```python
from build123d import *
from OCP.BRepFilletAPI import BRepFilletAPI_MakeChamfer

# Parameters (mm, degrees)
ESBO_O10_W               = 40
ESBO_O10_H               = 17.5
RESSALTO_EXTRUS_O6_DEPTH = 1.5
CORTE_EXTRUS_O2_DEPTH    = 2.5
ESBO_O12_W               = 3.5
ESBO_O12_H               = 2.75
RESSALTO_EXTRUS_O7_DEPTH = 1.2
ESBO_O13_W               = 3
ESBO_O13_H               = 1.5
ESBO_O13_W_2             = 2
CORTE_EXTRUS_O3_DEPTH    = 8
CORTE_EXTRUS_O4_DEPTH    = 20
CHANFRO5_SIZE            = 6
CHANFRO5_SIZE_2          = 0.419560872
CHANFRO6_SIZE            = 1
CHANFRO6_SIZE2           = 0.839099631
FILETE1_R                = 2


with BuildPart() as part:
    # Esboço10 → Ressalto-extrusão6 (new body)
    with BuildSketch(Plane.XY):
        Rectangle(ESBO_O10_W, ESBO_O10_H)
    extrude(amount=RESSALTO_EXTRUS_O6_DEPTH)

    # Esboço11 → Corte-extrusão2 (cut)
    with BuildSketch(Plane.XY.offset(1.5)):
        Polygon((-20, 3.75), (-15.75, 3.75), (-15.75, 8.75), (-12.25, 8.75), (-12.25, 3.75), (-3.75, 3.75), (-3.75, 9.75), (3.75, 9.75), (3.75, 3.75), (12.25, 3.75), (12.25, 8.75), (15.75, 8.75), (15.75, 3.75), (20, 3.75), (20, 11.902365005), (-20, 11.902365005), align=None)
        Polygon((-20, -4.25), (-15.75, -4.25), (-15.75, -8.75), (-12.25, -8.75), (-12.25, -4.25), (-3.75, -4.25), (-3.75, -10.25), (3.75, -9.74672567), (3.75, -4.25), (12.25, -4.25), (12.25, -8.75), (15.75, -8.75), (15.75, -4.25), (20, -4.25), (20, -11.31917021), (-20, -11.31917021), align=None)
    extrude(amount=-CORTE_EXTRUS_O2_DEPTH, mode=Mode.SUBTRACT)

    # Esboço12 → Ressalto-extrusão7 (add)
    with BuildSketch(Plane.XY.offset(1.5)):
        with Locations((-14, 7.375)):
            Rectangle(ESBO_O12_W, ESBO_O12_H)
        with Locations((-14, -7.375)):
            Rectangle(ESBO_O12_W, ESBO_O12_H)
        with Locations((14, -7.375)):
            Rectangle(ESBO_O12_W, ESBO_O12_H)
        with Locations((14, 7.375)):
            Rectangle(ESBO_O12_W, ESBO_O12_H)
    extrude(amount=RESSALTO_EXTRUS_O7_DEPTH)

    # Esboço13 → Corte-extrusão3 (cut)
    with BuildSketch(Plane.XY.offset(1.5)):
        with Locations((-10.75, 3)):
            Rectangle(ESBO_O13_W, ESBO_O13_H)
        with Locations((-5.25, 3)):
            Rectangle(ESBO_O13_W, ESBO_O13_H)
        with Locations((5.25, 3)):
            Rectangle(ESBO_O13_W, ESBO_O13_H)
        with Locations((10.75, 3)):
            Rectangle(ESBO_O13_W, ESBO_O13_H)
        with Locations((10.75, -3.5)):
            Rectangle(ESBO_O13_W, ESBO_O13_H)
        with Locations((5.25, -3.5)):
            Rectangle(ESBO_O13_W, ESBO_O13_H)
        with Locations((-5.25, -3.5)):
            Rectangle(ESBO_O13_W, ESBO_O13_H)
        with Locations((-10.75, -3.5)):
            Rectangle(ESBO_O13_W, ESBO_O13_H)
        with Locations((-16.75, -3.5)):
            Rectangle(ESBO_O13_W_2, ESBO_O13_H)
        with Locations((-16.75, 3)):
            Rectangle(ESBO_O13_W_2, ESBO_O13_H)
        with Locations((16.75, 3)):
            Rectangle(ESBO_O13_W_2, ESBO_O13_H)
        with Locations((16.75, -3.5)):
            Rectangle(ESBO_O13_W_2, ESBO_O13_H)
    extrude(amount=-CORTE_EXTRUS_O3_DEPTH, mode=Mode.SUBTRACT)

    # Esboço15 → Corte-extrusão4 (cut)
    with BuildSketch(Plane.XY.offset(1.5)):
        Polygon((-1.75, 5.75), (1.75, 5.75), (1.75, -5.75), (0, -7.015048633), (-1.75, -5.75), align=None)
    extrude(amount=-CORTE_EXTRUS_O4_DEPTH, mode=Mode.SUBTRACT)

    # Chanfro5
    chanfro5_edges_1 = [part.edges().sort_by_distance(p)[0] for p in [
        (-15.75, -8.75, 1.35),
    ]]
    chanfro5_side_1 = [part.faces().sort_by_distance(p)[0] for p in [
        (-15.75, -8.741608783, 1.35),
    ]]
    chanfro5_edges_2 = [part.edges().sort_by_distance(p)[0] for p in [
        (-3.75, -8.75, 0.75),
    ]]
    chanfro5_side_2 = [part.faces().sort_by_distance(p)[0] for p in [
        (-3.75, -8.741608783, 0.75),
    ]]
    chanfro5_edges_3 = [part.edges().sort_by_distance(p)[0] for p in [
        (12.25, -8.75, 1.35),
    ]]
    chanfro5_side_3 = [part.faces().sort_by_distance(p)[0] for p in [
        (12.25, -8.741608783, 1.35),
    ]]
    chanfro5_edges_4 = [part.edges().sort_by_distance(p)[0] for p in [
        (15.75, 8.75, 1.35),
    ]]
    chanfro5_side_4 = [part.faces().sort_by_distance(p)[0] for p in [
        (15.741608783, 8.75, 1.35),
    ]]
    chanfro5_edges_5 = [part.edges().sort_by_distance(p)[0] for p in [
        (3.75, 8.75, 0.75),
    ]]
    chanfro5_side_5 = [part.faces().sort_by_distance(p)[0] for p in [
        (3.741608783, 8.75, 0.75),
    ]]
    chanfro5_edges_6 = [part.edges().sort_by_distance(p)[0] for p in [
        (-12.25, 8.75, 1.35),
    ]]
    chanfro5_side_6 = [part.faces().sort_by_distance(p)[0] for p in [
        (-12.258391217, 8.75, 1.35),
    ]]
    chanfro5_edges_7 = [part.edges().sort_by_distance(p)[0] for p in [
        (-12.25, -8.75, 1.35),
    ]]
    chanfro5_side_7 = [part.faces().sort_by_distance(p)[0] for p in [
        (-12.258391217, -8.75, 1.35),
    ]]
    chanfro5_edges_8 = [part.edges().sort_by_distance(p)[0] for p in [
        (3.75, -8.75, 0.75),
    ]]
    chanfro5_side_8 = [part.faces().sort_by_distance(p)[0] for p in [
        (3.741608783, -8.75, 0.75),
    ]]
    chanfro5_edges_9 = [part.edges().sort_by_distance(p)[0] for p in [
        (15.75, -8.75, 1.35),
    ]]
    chanfro5_side_9 = [part.faces().sort_by_distance(p)[0] for p in [
        (15.741608783, -8.75, 1.35),
    ]]
    chanfro5_edges_10 = [part.edges().sort_by_distance(p)[0] for p in [
        (12.25, 8.75, 1.35),
    ]]
    chanfro5_side_10 = [part.faces().sort_by_distance(p)[0] for p in [
        (12.25, 8.741608783, 1.35),
    ]]
    chanfro5_edges_11 = [part.edges().sort_by_distance(p)[0] for p in [
        (-3.75, 8.75, 0.75),
    ]]
    chanfro5_side_11 = [part.faces().sort_by_distance(p)[0] for p in [
        (-3.75, 8.741608783, 0.75),
    ]]
    chanfro5_edges_12 = [part.edges().sort_by_distance(p)[0] for p in [
        (-15.75, 8.75, 1.35),
    ]]
    chanfro5_side_12 = [part.faces().sort_by_distance(p)[0] for p in [
        (-15.741608783, 8.75, 1.35),
    ]]
    chanfro5 = BRepFilletAPI_MakeChamfer(part.part.solid().wrapped)
    for e in chanfro5_edges_1:
        chanfro5.Add(CHANFRO5_SIZE - 0.0001, CHANFRO5_SIZE_2 - 0.0001, e.wrapped, chanfro5_side_1[0].wrapped)
    for e in chanfro5_edges_2:
        chanfro5.Add(CHANFRO5_SIZE - 0.0001, CHANFRO5_SIZE_2 - 0.0001, e.wrapped, chanfro5_side_2[0].wrapped)
    for e in chanfro5_edges_3:
        chanfro5.Add(CHANFRO5_SIZE - 0.0001, CHANFRO5_SIZE_2 - 0.0001, e.wrapped, chanfro5_side_3[0].wrapped)
    for e in chanfro5_edges_4:
        chanfro5.Add(CHANFRO5_SIZE_2 - 0.0001, CHANFRO5_SIZE - 0.0001, e.wrapped, chanfro5_side_4[0].wrapped)
    for e in chanfro5_edges_5:
        chanfro5.Add(CHANFRO5_SIZE_2 - 0.0001, CHANFRO5_SIZE - 0.0001, e.wrapped, chanfro5_side_5[0].wrapped)
    for e in chanfro5_edges_6:
        chanfro5.Add(CHANFRO5_SIZE_2 - 0.0001, CHANFRO5_SIZE - 0.0001, e.wrapped, chanfro5_side_6[0].wrapped)
    for e in chanfro5_edges_7:
        chanfro5.Add(CHANFRO5_SIZE_2 - 0.0001, CHANFRO5_SIZE - 0.0001, e.wrapped, chanfro5_side_7[0].wrapped)
    for e in chanfro5_edges_8:
        chanfro5.Add(CHANFRO5_SIZE_2 - 0.0001, CHANFRO5_SIZE - 0.0001, e.wrapped, chanfro5_side_8[0].wrapped)
    for e in chanfro5_edges_9:
        chanfro5.Add(CHANFRO5_SIZE_2 - 0.0001, CHANFRO5_SIZE - 0.0001, e.wrapped, chanfro5_side_9[0].wrapped)
    for e in chanfro5_edges_10:
        chanfro5.Add(CHANFRO5_SIZE - 0.0001, CHANFRO5_SIZE_2 - 0.0001, e.wrapped, chanfro5_side_10[0].wrapped)
    for e in chanfro5_edges_11:
        chanfro5.Add(CHANFRO5_SIZE - 0.0001, CHANFRO5_SIZE_2 - 0.0001, e.wrapped, chanfro5_side_11[0].wrapped)
    for e in chanfro5_edges_12:
        chanfro5.Add(CHANFRO5_SIZE_2 - 0.0001, CHANFRO5_SIZE - 0.0001, e.wrapped, chanfro5_side_12[0].wrapped)
    add(Compound.cast(chanfro5.Shape()), mode=Mode.REPLACE)  # a hair under: the kernel refuses the full size

    # Chanfro6: one chamfer whose edges measure the first distance from different faces: ONE call of the kernel's chamfer builder (chamfer() names one face for all edges)
    chanfro6_edges_1 = [part.edges().sort_by_distance(p)[0] for p in [
        (0, -8.75, 1.5),
    ]]
    chanfro6_side_1 = [part.faces().sort_by_distance(p)[0] for p in [
        (0, -8.75, 0.75),
    ]]
    chanfro6_edges_2 = [part.edges().sort_by_distance(p)[0] for p in [
        (0, 8.75, 1.5),
    ]]
    chanfro6_side_2 = [part.faces().sort_by_distance(p)[0] for p in [
        (0, 8.75, 0.75),
    ]]
    chanfro6 = BRepFilletAPI_MakeChamfer(part.part.solid().wrapped)
    for e in chanfro6_edges_1:
        chanfro6.Add(CHANFRO6_SIZE, CHANFRO6_SIZE2, e.wrapped, chanfro6_side_1[0].wrapped)  # the first distance lies on this face
    for e in chanfro6_edges_2:
        chanfro6.Add(CHANFRO6_SIZE, CHANFRO6_SIZE2, e.wrapped, chanfro6_side_2[0].wrapped)  # the first distance lies on this face
    add(Compound.cast(chanfro6.Shape()), mode=Mode.REPLACE)

    # Filete1
    filete1_edges = [part.edges().sort_by_distance(p)[0] for p in [
        (-14, -8.75, 2.7),
        (14, -8.75, 2.7),
        (14, 8.75, 2.7),
        (-14, 8.75, 2.7),
    ]]
    fillet(filete1_edges, radius=FILETE1_R)


solid = part.part
```
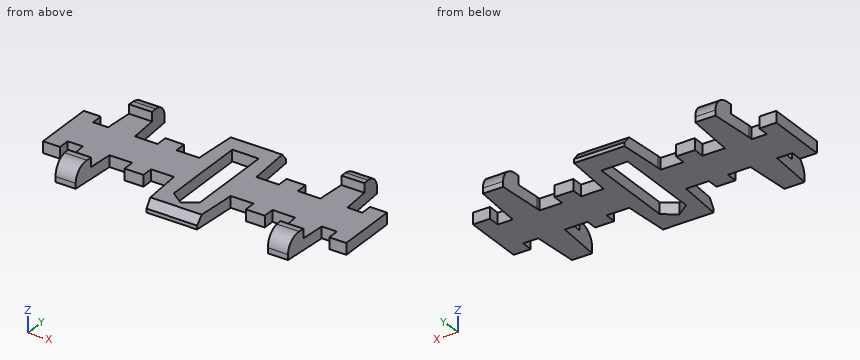
Build history of the part. All positions in model axes, mm. Coordinates: 2 decimals unless noted, no trailing zeros. Order: outer loops, then holes, each group sorted by start corner. A loop starts at its lowest first (then second) coordinate and runs counter-clockwise, first axis right, second up. Notation, with made-up numbers: (-10, 6.5) -> (25, 6.5) arc R18 cw to (25, 37.5) -> close; hole circle Ø11 at (64.25, -1.75). An arc over 180 degrees is marked (long way). Answer in a Markdown table with one row per item. Add a question column.
Q1. Band-saw the part on C-C, the plane x = 1. List the corners of the cut face in (y, z).
Q2. Band-saw the part on B-B, the plane y = 0.75. List the corners of the cut face in (x, z), then the cut area to 4 significant figures.
Q3. Band-saw the part on D-D, the plane y = 4.25. List the corners of the cut face in (x, z), then the cut area to 3 significant figures.
Q4. Wall check: line 1 along X through (y, z) = (2, 0.2); line 2 along X through (y, z) = (5.25, 0.8); line 3 along Z through (x, y) = (11.5, -2). Give the ranges that are in metal, low to high. Write a range as [from, to].
Q5. Drop flat-ended pins along their axis: pin 1 (1 mm diameter, centred on y = 5, z = 1.5, fed in from +X); pin 2 (1 mm diameter, centred on x = -10.5, z = 1.5, fed in from +Y); pin 3 (1.2 mm diameter, centred on x = -7.5, z = 0.5, fed in from +Y). Give the stop position or say it passes through.
Q6. Band-saw the part on A-A, the plane z = 1.85. List the corners of the cut face in (x, y), then the cut area to 3 significant figures.
Answers follow:
| question | item | result |
|---|---|---|
| 1 | outline | (-8.75, 0) -> (-6.29, 0) -> (-6.29, 1.5) -> (-7.91, 1.5) -> (-8.75, 0.5) -> close; (5.75, 0) -> (8.75, 0) -> (8.75, 0.5) -> (7.91, 1.5) -> (5.75, 1.5) -> close |
| 2 | outline | (-20, 0) -> (-1.75, 0) -> (-1.75, 1.5) -> (-20, 1.5) -> close; (1.75, 0) -> (20, 0) -> (20, 1.5) -> (1.75, 1.5) -> close |
| 2 | area | 54.75 mm^2 |
| 3 | outline | (-15.65, 0) -> (-12.35, 0) -> (-12.35, 1.5) -> (-15.65, 1.5) -> close; (-3.65, 0) -> (-1.75, 0) -> (-1.75, 1.5) -> (-3.65, 1.5) -> close; (1.75, 0) -> (3.65, 0) -> (3.65, 1.5) -> (1.75, 1.5) -> close; (12.35, 0) -> (15.65, 0) -> (15.65, 1.5) -> (12.35, 1.5) -> close |
| 3 | area | 15.6 mm^2 |
| 4 | line 1 | [-20, -1.75], [1.75, 20] |
| 4 | line 2 | [-15.58, -12.42], [-3.58, -1.75], [1.75, 3.58], [12.42, 15.58] |
| 4 | line 3 | [0, 1.5] |
| 5 | pin 1 | x = 15.63 |
| 5 | pin 2 | y = 2.25 |
| 5 | pin 3 | y = 3.75 |
| 6 | outline | (-15.52, -6) -> (-15.36, -8.39) -> (-12.64, -8.39) -> (-12.48, -6) -> close; (-15.52, 6) -> (-12.48, 6) -> (-12.64, 8.39) -> (-15.36, 8.39) -> close; (12.48, -6) -> (12.64, -8.39) -> (15.36, -8.39) -> (15.52, -6) -> close; (12.48, 6) -> (15.52, 6) -> (15.36, 8.39) -> (12.64, 8.39) -> close |
| 6 | area | 27.5 mm^2 |
